from build123d import *

# Parameters (mm, degrees)
F0_W     = 87
F0_H     = 71
F1_DEPTH = 20
F2_W     = 2.5
F2_H     = 10
F3_DEPTH = 13.5
F4_R     = 8
F5_W     = 23
F5_H     = 17
F5_W_2   = 39
F5_R     = 4.75
F5_R_2   = 2
F5_R_3   = 2.5
F6_DEPTH = 17


with BuildPart() as f1:
    # F0 (on Top) → F1 (new body)
    with BuildSketch(Plane.XY):
        Rectangle(F0_W, F0_H)
    extrude(amount=F1_DEPTH)

    # F2 (on face) → F3 (cut)
    with BuildSketch(Plane(origin=(0, 0, 0), x_dir=(1, 0, 0), z_dir=(0, 0, -1))):
        with Locations((-15.25, 30.5)):
            Rectangle(F2_W, F2_H)
        with Locations((15.25, 30.5)):
            Rectangle(F2_W, F2_H)
        with Locations((-15.25, -30.5)):
            Rectangle(F2_W, F2_H)
        with Locations((15.25, -30.5)):
            Rectangle(F2_W, F2_H)
    extrude(amount=-F3_DEPTH, mode=Mode.SUBTRACT)

    # F4
    f4_edges = [f1.edges().sort_by_distance(p)[0] for p in [
        (-43.5, 0, 0),
    ]]
    fillet(f4_edges, radius=F4_R)

    # F5 (on face) → F6 (cut)
    with BuildSketch(Plane.XY.offset(20)):
        with Locations((-29, -24)):
            Rectangle(F5_W, F5_H)
        with Locations((21, -24)):
            Rectangle(F5_W_2, F5_H)
        with Locations((-7.390061, -24)):
            Circle(F5_R)
        with Locations((-38.5, -8.499949)):
            Circle(F5_R_2)
        with Locations((-29.5, -8.499949)):
            Circle(F5_R_2)
        with Locations((-20.5, -8.499949)):
            Circle(F5_R_2)
        with Locations((-11.5, -8.499949)):
            Circle(F5_R_2)
        with Locations((-2.5, -8.499949)):
            Circle(F5_R_2)
        with Locations((7, -8.499949)):
            Circle(F5_R_3)
        with Locations((17, -8.499949)):
            Circle(F5_R_3)
        with Locations((27, -8.499949)):
            Circle(F5_R_3)
        with Locations((37, -8.499949)):
            Circle(F5_R_3)
        with Locations((37.5, 1.500051)):
            Circle(F5_R_2)
        with Locations((30, 1.500051)):
            Circle(F5_R_2)
        with Locations((22.5, 1.500051)):
            Circle(F5_R_2)
        with Locations((15, 1.500051)):
            Circle(F5_R_2)
        with Locations((7.5, 1.500051)):
            Circle(F5_R_2)
        with Locations((0, 1.500051)):
            Circle(F5_R_2)
        with Locations((-7.5, 1.500051)):
            Circle(F5_R_2)
        with Locations((-20.5, 1.500051)):
            Circle(F5_R_2)
        with Locations((-34.5, 1.500051)):
            Circle(F5_R_2)
        with Locations((-34.460917, 11.500051)):
            Circle(F5_R_2)
        with Locations((-34.5, 26.5)):
            Circle(F5_R_2)
        with Locations((-17.5, 26.5)):
            Circle(F5_R_2)
        with Locations((-17.460917, 11.500051)):
            Circle(F5_R_2)
        with Locations((-0.460917, 11.500051)):
            Circle(F5_R_2)
        with Locations((-0.5, 26.5)):
            Circle(F5_R_2)
        with Locations((16.5, 26.5)):
            Circle(F5_R_2)
        with Locations((16.539083, 11.500051)):
            Circle(F5_R_2)
        with Locations((33.539083, 11.500051)):
            Circle(F5_R_2)
        with Locations((33.5, 26.5)):
            Circle(F5_R_2)
    extrude(amount=-F6_DEPTH, mode=Mode.SUBTRACT)


solid = f1.part
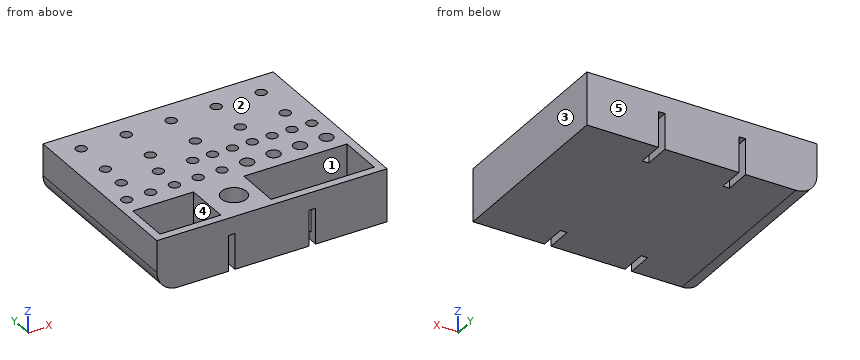
Build history of the part. All positions in model axes, mm. Face numbers are marked on the shaded views. A direction names the side the tool comes from. Give positions to 0.01 mm unless a question says otherwise; leave off trailing zeros. Order: outer loops, then holes, each group sorted by start corner. A loop starts at its lowest first (then second) coordinate and runs counter-clockwise, first axis right, second up. Notation, with made-up numbers: M 84.25,5.5 L 129.25,5.5 A15 cw 129.25,15.5 Z; hole C 80.5,86 d4. An arc over 180 degrees is marked long. Use one line per item in the form item = value.
1) Drop a flat-ended pin along its axis: pin 1 (3 mm diameter, centred on x = -38.5, y = -8.5, fed in from +Z). Give the stop position or say it passes through.
Calculated:
pin_1 = 3
2) Saw through at B-B (y = -24). Give the cut face in (x, z).
Calculated:
outline = M -43.5,8 A8 ccw -35.5,0 L 43.5,0 L 43.5,20 L 40.5,20 L 40.5,3 L 1.5,3 L 1.5,20 L -2.64,20 L -2.64,3 L -12.14,3 L -12.14,20 L -17.5,20 L -17.5,3 L -40.5,3 L -40.5,20 L -43.5,20 Z
3) Saw through at A-A (x = -29.5). Give the cut face in (y, z).
Calculated:
outline = M -35.5,0 L 35.5,0 L 35.5,20 L -6.5,20 L -6.5,3 L -10.5,3 L -10.5,20 L -15.5,20 L -15.5,3 L -32.5,3 L -32.5,20 L -35.5,20 Z
4) Two-plate mould, pull along X, no slides. Class the marked faces 1, 2 and 3: released by +X, released by -X, zero draft, split by the parting line, or undercut.
Calculated:
face_1 = undercut
face_2 = zero draft
face_3 = released by +X
5) Saw through at C-C (x = 11.5). Give the cut face in (y, z).
Calculated:
outline = M -35.5,0 L 35.5,0 L 35.5,20 L -15.5,20 L -15.5,3 L -32.5,3 L -32.5,20 L -35.5,20 Z
6) Saw through at D-D (z = 15.5). State how many separate pieces and enclosed holes the cut face has, plus the area to 3 significant figures.
Calculated:
separate_pieces = 1
enclosed_holes = 31
area = 4,670 mm2
7) Tool access for the marked faces 4 and 5: list every direction of +Z, -Z, +X, -X, +Y, -Y with a clear straight run to the whole face (end or side of a thin tool).
Calculated:
face_4 = +Z
face_5 = +Z, -Z, +X, -X, +Y
8) Probe probe 1 along Y at (x, z) = (4, 6); probe 2 along Y at (x, z) = (36, 3.5); probe 3 along Y at (x, z) = (7.5, 13). List the from-to ranges inside material, lowest first.
Calculated:
probe_1 = -35.5 to -32.5, -15.5 to 35.5
probe_2 = -35.5 to -32.5, -15.5 to -10.79, -6.21 to 0.18, 2.82 to 35.5
probe_3 = -35.5 to -32.5, -15.5 to -10.95, -6.05 to -0.5, 3.5 to 35.5
